The model under review builds one solid part; all positions refer to its coordinate system, in mm. A direction names the side the tool comes from. Coordinates: 2 decimals unless noted, no trailing zeros. Loops run counter-clockwise (first coordinate to the right, second up) from the corner with the lowest first, then second, coordinate; pieces in that order, holes last. Notation, with made-up numbers: M 33,-26 L 41,-26 A31 cw 41,5 Z; hole C -27,3.5 d10. An arc over 180 degrees is marked long. One line per item, written item: value.
```python
from build123d import *

# Parameters (mm, degrees)
SKETCH1_R           = 57.15
BOSS_EXTRUDE1_DEPTH = 38.1
SKETCH2_R           = 25.4
CUT_EXTRUDE1_DEPTH  = 38.1
SKETCH3_R           = 50.8
CUT_EXTRUDE2_DEPTH  = 7.62
CUT_EXTRUDE3_START  = -7.62
SKETCH5_R           = 50.8
CUT_EXTRUDE3_DEPTH  = 7.62


with BuildPart() as part:
    # Sketch1 → Boss-Extrude1 (new body)
    with BuildSketch(Plane.XY):
        with Locations(Location((0, 0, 0), (0, 0, 180))):
            Circle(SKETCH1_R)
    extrude(amount=BOSS_EXTRUDE1_DEPTH)

    # Sketch2 → Cut-Extrude1 (cut)
    with BuildSketch(Plane.XY.offset(38.1)):
        Circle(SKETCH2_R)
    extrude(amount=-CUT_EXTRUDE1_DEPTH, mode=Mode.SUBTRACT)

    # Sketch3 → Cut-Extrude2 (cut)
    with BuildSketch(Plane.XY.offset(38.1)):
        Circle(SKETCH3_R)
    extrude(amount=-CUT_EXTRUDE2_DEPTH, mode=Mode.SUBTRACT)

    # Sketch5 → Cut-Extrude3 (cut)
    with BuildSketch(Plane(origin=(0, 0, 0), x_dir=(-1, 0, 0), z_dir=(0, 0, -1)).offset(CUT_EXTRUDE3_START)):
        with Locations(Location((0, 0, 0), (0, 0, 180))):
            Circle(SKETCH5_R)
    extrude(amount=CUT_EXTRUDE3_DEPTH, mode=Mode.SUBTRACT)


solid = part.part
```
(1) Insertion check: pin 1 Ø12 at (x, y) = (40.5, -17) entering from -Z; pin 2 Ø6 at (x, y) = (4.5, 20) entering from +Z; pin 3 Ø4 at (x, z) = (6, 31) entering from -Y; pin 4 Ø10 at (x, z) = (15, 19.5) entering from +Y. Each pin has a flat end and moves straight along its axis. Give the tip position at first contact, or say it passes through.
Checks:
pin 1: z = 7.62
pin 2: through
pin 3: y = -57.01
pin 4: y = 56.27
(2) Draft analysis for pull direction X (two halves, no side actions). For faces 4 (the face through (10.6, -23.3, 7.62)), 5 (the face through (38, 34, 38.1)), 6 (the face through (57.095, -2.513, 18.783)), state which applies: pulls with the +X half, pulls with the -X half, needs draft (parallel to the pull), parting line crosses it, or undercut.
Checks:
face 4: undercut
face 5: needs draft
face 6: parting line crosses it
(3) Add section A-A on y = 0. State the section outline as (x, z) points, then the cut area to 3 significant figures.
Checks:
outline: M -57.15,0 L -50.8,0 L -50.8,7.62 L -25.4,7.62 L -25.4,30.48 L -50.8,30.48 L -50.8,38.1 L -57.15,38.1 Z; M 25.4,7.62 L 50.8,7.62 L 50.8,0 L 57.15,0 L 57.15,38.1 L 50.8,38.1 L 50.8,30.48 L 25.4,30.48 Z
area: 1,650 mm^2
(4) Tool access review of faces 1 (the face through (23.44, 45.07, 3.86)), 2 (the face through (10.6, 23.3, 30.48)), 3 (the face through (-5.506, -24.796, 19.21)): name each direction out of +Z, -Z, +X, -X, +Y, -Y from which nothing blocks a thin tool from reaching the whole face with its end or side.
Checks:
face 1: -Z
face 2: +Z
face 3: +Z, -Z
(5) To check wall thickness, follow L1, parallel to Y at x = 0, z = 24; L2, parallel to Y at x = 0, z = 36; L3, parallel to X at y = -1.5, z = 32. State the ranges of each line that lie inside material, in increasing order. Write a range as [from, to].
Checks:
L1: [-57.15, -25.4], [25.4, 57.15]
L2: [-57.15, -50.8], [50.8, 57.15]
L3: [-57.13, -50.78], [50.78, 57.13]
(6) Add section D-D on x = -41.5. State the section outline as (y, z) points, then the cut area to 3 significant figures.
Checks:
outline: M -39.29,0 L -29.3,0 L -29.3,7.62 L 29.3,7.62 L 29.3,0 L 39.29,0 L 39.29,38.1 L 29.3,38.1 L 29.3,30.48 L -29.3,30.48 L -29.3,38.1 L -39.29,38.1 Z
area: 2,100 mm^2
(7) Add section C-C on z = 22.5. State the section outline as (x, y) points.
Checks:
outline: C 0,0 d114.3; hole C 0,0 d50.8
